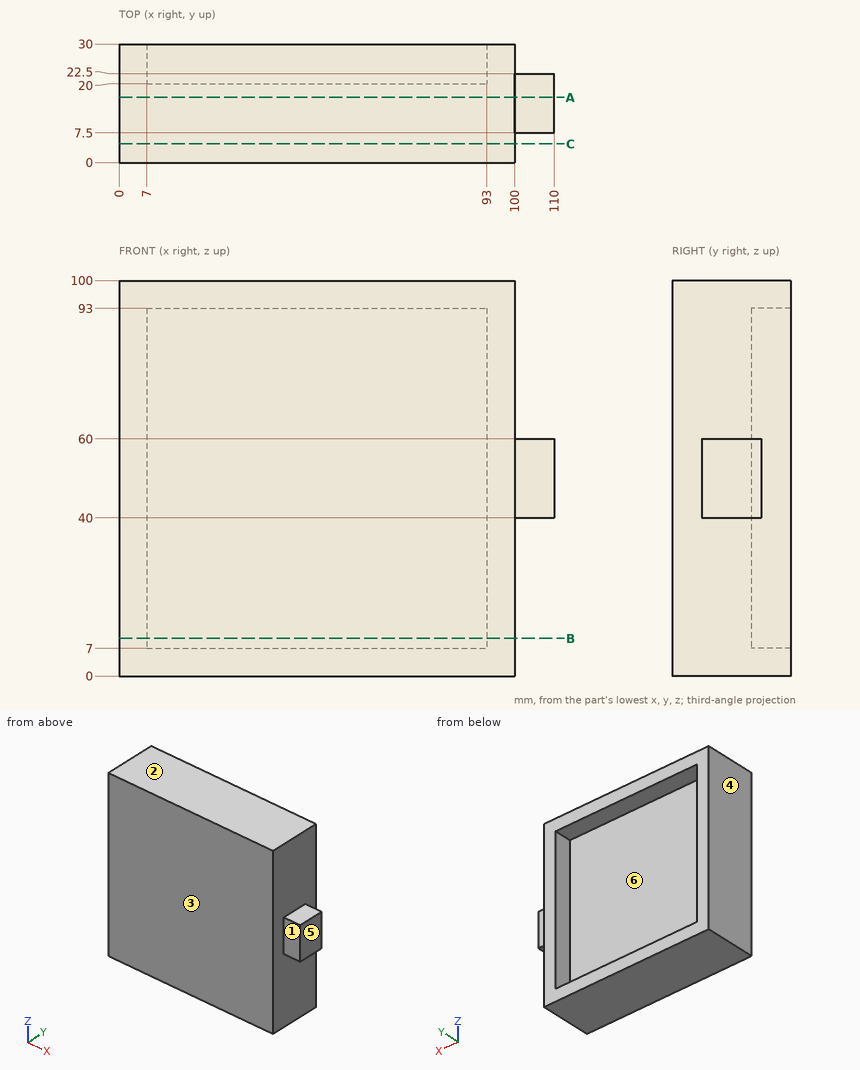
Geometry check sheet. Reference: drawing and pictorial views, mm from the part's lowest x, y, z. A direction names the side the tool comes from. Give positions to 0.01 mm unless a question says otherwise; leave off trailing zeros. Write each loop counter-clockwise with the first axis right and the second up, starting at its lowest first coordinate (ties: lowest second). Pieces come first, ordered by that corner, then holes. Notation, with made-up numbers: M -37.75,-28 L -16.75,-28 A18 ccw -16.75,-5 Z; hole C 80,40.5 d2. An arc over 180 degrees is marked long. Put each result on its own line as item: value. Start each with the question number.
1. Draft check along X on the marked faces 3, 4, 5 and 6. Enter one of: +X half, -X half, draft (parallel to the pull), parting line (faces both ways), or undercut.
2. Section check B-B (z = 9.5). Record the cut outline in (x, y).
3. Go/stop test with flat-tipped pins: pin 1 Ø11 at (y, z) = (24.5, 71.5) entering from +X; pin 2 Ø11 at (x, z) = (106.5, 52) entering from -Y; pin 3 Ø5 at (x, z) = (84.5, 57.5) entering from -Y; pin 4 Ø3 at (x, y) = (103, 12.5) entering from +Z. Record where each tip stops, or that it passes through.
4. Section check C-C (y = 4.75). Record the cut outline in (x, z), and give its area (3 significant figures).
5. Section check A-A (y = 16.5). Record the cut outline in (x, z), and give its area (3 significant figures).
6. Scan lines: line 1 along X through (y, z) = (21.25, 85.5); line 2 along X through (y, z) = (15.75, 26). Record each from-to range of solid material in increasing order. Write a range as [from, to].
7. Set-up check for the marked faces 1 and 2: record each of +Z, -Z, +X, -X, +Y, -Y from which the full face is reachable in a straight line by a thin tool's end or side.
Answer list:
1. face 3: draft
1. face 4: -X half
1. face 5: +X half
1. face 6: undercut
2. outline: M 0,0 L 100,0 L 100,30 L 93,30 L 93,20 L 7,20 L 7,30 L 0,30 Z
3. pin 1: x = 100
3. pin 2: y = 7.5
3. pin 3: y = 0
3. pin 4: z = 60
4. outline: M 0,0 L 100,0 L 100,100 L 0,100 Z
4. area: 10,000 mm2
5. outline: M 0,0 L 100,0 L 100,40 L 110,40 L 110,60 L 100,60 L 100,100 L 0,100 Z
5. area: 10,200 mm2
6. line 1: [0, 7], [93, 100]
6. line 2: [0, 100]
7. face 1: +Z, -Z, +X, -Y
7. face 2: +Z, +X, -X, +Y, -Y
